Job drawing, mm, ordinate dimensions from the low corner. One solid piece. A direction names the side the tool comes from. Round coordinates to 2 decimals unless told otherwise and drop trailing zeros. Write each loop counter-clockwise with the first axis right and the second up, starting at its lowest first coordinate (ties: lowest second). Pieces come first, ordered by that corner, then holes. Notation, with made-up numbers: (-32.5, 77) -> (1.5, 77) arc R9 ccw to (1.5, 86) -> close; hole circle Ø8 at (55, -21.75). An arc over 180 degrees is marked (long way). Use CSV: the item, a comma, the result in double quotes. Start each with the question number.
(1) Saw through at A-A (x = 120). Give the cut face in (y, z), plus the area to 3 significant figures.
(2) Saw through at B-B (z = 8). Give the cut face in (x, y), plus the area to 3 significant figures.
(3) Probe line 1 (Y direction, x = 120, z = 7); line 2 (X direction, y = 42, z = 8.25); line 3 (Y direction, x = 20, z = 4.75). List the from-to ranges inside material, lowest first. Write a range as [from, to].
(4) Two-plate mould, pull along Y, no slides. Class the marked faces 1, 2, 3 and 4: released by +Y, released by -Y, zero draft, split by the parting line, or undercut.
(5) Drop flat-ended pins along their axis: pin 1 (3 mm diameter, centred on x = 80, z = 7.5, fed in from +Y); pin 2 (5 mm diameter, centred on y = 40.5, z = 3, fed in from -X); pin 3 (3 mm diameter, centred on x = 54, z = 2.5, fed in from +Y); pin 4 (24 mm diameter, centred on x = 120, y = 57.59, fed in from +Z). Give the stop position or say it passes through.
(6) Saw through at C-C (y = 27). Give the cut face in (x, z).
(7) Saw through at D-D (x = 139.5). Give the cut face in (y, z).
(8) Which spindle directions (+Z, -Z, +X, -X, +Y, -Y) get a long thin tool onto all of the face, cutting with end or side? Do the marked faces 5, 6 and 7. Say none if no direction does.
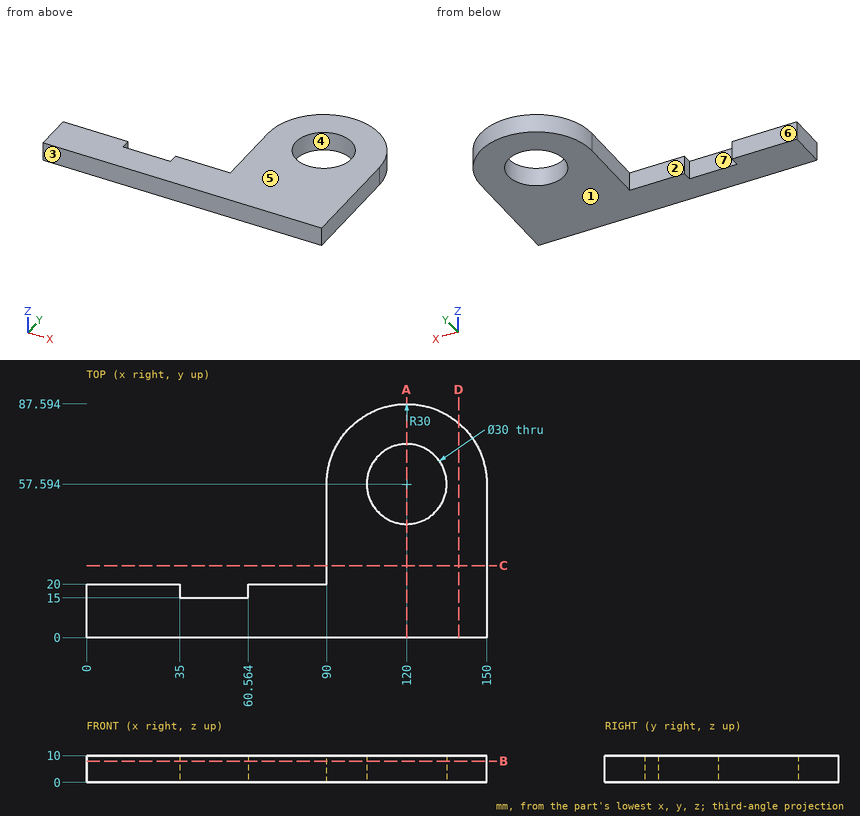
Answers:
1,outline,"(0, 0) -> (42.59, 0) -> (42.59, 10) -> (0, 10) -> close; (72.59, 0) -> (87.59, 0) -> (87.59, 10) -> (72.59, 10) -> close"
1,area,"576 mm²"
2,outline,"(0, 0) -> (150, 0) -> (150, 57.59) arc R30 ccw to (90, 57.59) -> (90, 20) -> (60.56, 20) -> (60.56, 15) -> (35, 15) -> (35, 20) -> (0, 20) -> close; hole circle Ø30 at (120, 57.59)"
2,area,"5,830 mm²"
3,line 1,"y = [0, 42.59], [72.59, 87.59]"
3,line 2,"x = [90, 150]"
3,line 3,"y = [0, 20]"
4,face 1,"zero draft"
4,face 2,"released by +Y"
4,face 3,"released by -Y"
4,face 4,"undercut"
5,pin 1,"stops at y = 20"
5,pin 2,"stops at x = 90"
5,pin 3,"stops at y = 15"
5,pin 4,"passes through"
6,outline,"(90, 0) -> (150, 0) -> (150, 10) -> (90, 10) -> close"
7,outline,"(0, 0) -> (80.39, 0) -> (80.39, 10) -> (0, 10) -> close"
8,face 5,"+Z, +X, -X, +Y, -Y"
8,face 6,"+Z, -Z, -X, +Y"
8,face 7,"+Z, -Z, +Y"
